For this review, use the dimensioned drawing (mm, ordinates from the lowest corner) and the shaded views. Round coordinates to 2 decimals unless told otherwise and drop trailing zeros. Order: outer loops, then holes, each group sorted by start corner. A loop starts at its lowest first (then second) coordinate and runs counter-clockwise, first axis right, second up. Notation, with made-up numbers: M -27.75,-2 L 12.25,-2 A24 ccw 12.25,11 Z; hole C -3,-4 d6. An arc over 180 degrees is marked long. Put each result on its own line as item: value.
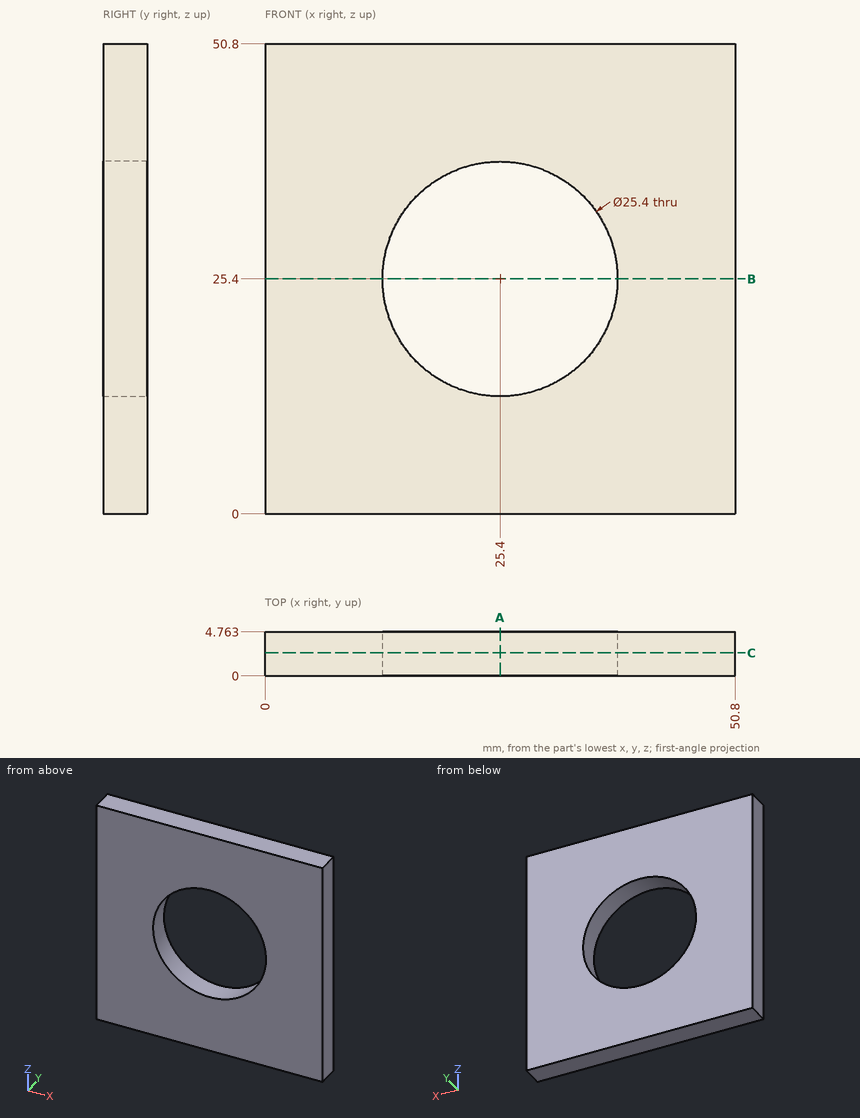
(1) Add section B-B on z = 25.4. Give the boundary of the cut face in (x, y), then the cut area to 3 significant figures.
A:
outline: M 0,0 L 12.7,0 L 12.7,4.76 L 0,4.76 Z; M 38.1,0 L 50.8,0 L 50.8,4.76 L 38.1,4.76 Z
area: 121 mm2
(2) Add section C-C on y = 2.5. Give the boundary of the cut face in (x, z).
A:
outline: M 0,0 L 50.8,0 L 50.8,50.8 L 0,50.8 Z; hole C 25.4,25.4 d25.4
(3) Add section A-A on x = 25.4. Give the boundary of the cut face in (y, z).
A:
outline: M 0,0 L 4.76,0 L 4.76,12.7 L 0,12.7 Z; M 0,38.1 L 4.76,38.1 L 4.76,50.8 L 0,50.8 Z
(4) To check wall thickness, follow L1, parallel to X at y = 2.85, z = 25.4; L2, parallel to X at y = 3.2, z = 37 (1 decimal). State the ranges of each line that lie inside material, in increasing order.
A:
L1: x = 0 to 12.7, 38.1 to 50.8
L2: x = 0 to 20.2, 30.6 to 50.8
